Input: part model. Units: mm. Frame: model coordinates. A direction names the side the tool comes from. Coordinates: 2 decimals unless noted, no trailing zeros. Order: outer loops, then holes, each group sorted by start corner. A loop starts at its lowest first (then second) coordinate and runs counter-clockwise, first axis right, second up. Notation, with made-up numbers: (-8, -10.75) - (35, -10.75) arc R20 cw to (35, 27.25) - close; hole circle Ø1 at (9.5, -29.75). An arc over 180 degrees is marked (long way). Use a Markdown table: item, result. Add a question column.
Solid Edge part; units mm, degrees
sketch "Sketch1" plane through (0, 0, 0) normal (0, 0, 1) x (1, 0, 0)
  line L0 (2.5, 0) -> (2.5, 12)
  line L1 (0, 12) -> (2.5, 12)
  line L2 (0, 0) -> (0, 12)
  line L3 (0, 0) -> (0, -2.75)
  line L4 (0, -2.75) -> (4.75, -2.75)
  line L5 (4.75, -2.75) -> (4.75, 0)
  line L6 (4.75, 0) -> (2.5, 0)
revolve "RevolvedProtrusion1" add sketch "Sketch1" angle 360 about axis through (0, 0, 0) along (0, 1, 0)
sketch "Sketch2" plane through (0, 0, 0) normal (1, 0, 0) x (0, 1, 0)
  line L0 (-2.75, 2.2215) -> (-1.19, 2.2215)
  line L1 (0.0926, 0) -> (-1.19, 2.2215)
  line L2 (-2.75, 0) -> (0.0926, 0)
  line L3 (-2.75, 0) -> (-2.75, 2.2215)
revolve "RevolvedCutout1" cut sketch "Sketch2" angle 360 about axis through (0, -4.5, 0) along (0, 1, 0)
sketch "Sketch3" plane through (0, -2.75, 0) normal (0, -1, 0) x (0, 0, 1)
  circle A0 centre (0, 0) radius 2.2215
  line L0 (-1.5, -0.866) -> (0, -1.7321)
  line L1 (0, -1.7321) -> (1.5, -0.866)
  line L2 (1.5, -0.866) -> (1.5, 0.866)
  line L3 (1.5, 0.866) -> (0, 1.7321)
  line L4 (0, 1.7321) -> (-1.5, 0.866)
  line L5 (-1.5, 0.866) -> (-1.5, -0.866)
extrude "Protrusion1" add sketch "Sketch3" against normal up to next
sketch "Sketch4" plane through (0, 0, 0) normal (0, 0, 1) x (1, 0, 0)
  line L0 (-1.7321, -2.75) -> (0, -2.75)
  line L1 (0, -2.75) -> (0, -2.2859)
  line L2 (0, -2.2859) -> (-1.7321, -2.75)
revolve "RevolvedCutout2" cut sketch "Sketch4" angle 360 about axis through (0, -4.5, 0) along (0, 1, 0)
fillet "Round1" radius 0.2 1 edges at (0, 0, -2.5)
chamfer "倒斜角_2" distance 0.3333 angle 45 1 edges at (0, 12, -2.5)
cosmetic_thread "螺纹_3" thread depth 10.4
sketch "Sketch5" plane through (0, 0, 0) normal (0, 0, 1) x (1, 0, 0)
  arc A0 (-2.2953, -2.75) -> (-4.75, 0) centre (-1.9822, 0) cw
revolve "RevolvedCutout3" cut sketch "Sketch5" angle 360 about axis through (0, 0, 0) along (0, -1, 0) material side at (-4.0844, -1.8764, 0)
1) Reachability of faces 4 (the flat face through (-1.293, -1.776, 0.76)), 5 (the flat face through (0, -2.75, -2)) from +Z, -Z, +X, -X, +Y, -Y: full face, straight path, thin tool, end or side. Return the list, or none.
2) Material intervals for L1, parallel to Z at x = 1, y = 9.5; L2, parallel to Y at x = 1.75, z = 2; L3, parallel to Z at x = 0, y = 0.25, sorted ascending.
3) Pull-direction query (X, two-part tool) for faces 1 (the flat face through (-1.305, -1.776, -0.739)), 2 (the flat face through (2.04, 0, 2.04)), 3 (the cylindrical face through (-0.54, 6.01, 2.44)); classes: pulls with the +X half, pulls with the -X half, needs draft (parallel to the pull), parting line crosses it, or undercut.
4) Contact query for flat-ended pins moving along their axis: P1, Ø0.5, axis at x = 0, y = -1.5, coming from the -Z side; P2, Ø4, axis at y = 1.5, z = 2.5, coming from the +X side; P3, Ø3, axis at y = 1, z = -1.5, coming from the -X side; P4, Ø3, axis at x = -1.5, z = 2, coming from the +Y side. Output: stop coordinate, or through.
5) Cut plane A-A (y = 9.75). Return the cut outline in (x, z).
Computed:
| question | item | result |
|---|---|---|
| 1 | face 4 | -Y |
| 1 | face 5 | +Z, -Z, +X, -X, -Y |
| 2 | L1 | z = -2.29 to 2.29 |
| 2 | L2 | y = -2.68 to 0 |
| 2 | L3 | z = -2.5 to 2.5 |
| 3 | face 1 | undercut |
| 3 | face 2 | needs draft |
| 3 | face 3 | parting line crosses it |
| 4 | P1 | stops at z = -4.45 |
| 4 | P2 | stops at x = 4.6 |
| 4 | P3 | stops at x = -4.73 |
| 4 | P4 | stops at y = 12 |
| 5 | outline | circle Ø5 at (0, 0) |
